```python
from build123d import *

# Parameters (mm, degrees)
F0_W      = 26
F0_H      = 26
F0_W_2    = 16
F0_H_2    = 16
F1_DEPTH  = 2
F2_DEPTH  = 100
F3_W      = 26
F3_H      = 26
F3_W_2    = 18
F3_H_2    = 18
F4_DEPTH  = 4
F5_W      = 5
F5_H      = 4
F6_DEPTH  = 4
F7_D      = 2.7
F7_DEPTH  = 4
F7_TIP    = 0.8111618357
F9_W      = 3
F9_H      = 16
F10_DEPTH = 26
F11_W     = 4
F11_H     = 12
F12_DEPTH = 20


with BuildPart() as f1:
    # F0 (on Top) → F1 (new body)
    with BuildSketch(Plane.XY):
        Rectangle(F0_W, F0_H)
        Rectangle(F0_W_2, F0_H_2, mode=Mode.SUBTRACT)
        Rectangle(F0_W_2, F0_H_2)
    extrude(amount=F1_DEPTH)

    # F0 (on Top) → F2 (join)
    with BuildSketch(Plane.XY):
        Rectangle(F0_W, F0_H)
        Rectangle(F0_W_2, F0_H_2, mode=Mode.SUBTRACT)
    extrude(amount=F2_DEPTH)

    # F3 (on face) → F4 (join)
    with BuildSketch(Plane.XY.offset(100)):
        Rectangle(F3_W, F3_H)
        Rectangle(F3_W_2, F3_H_2, mode=Mode.SUBTRACT)
    extrude(amount=F4_DEPTH)

    # F5 (on face) → F6 (cut, through all)
    with BuildSketch(Plane.XY.offset(104)):
        with Locations((0, -11)):
            Rectangle(F5_W, F5_H)
        with Locations((0, 11)):
            Rectangle(F5_W, F5_H)
    extrude(amount=-F6_DEPTH, mode=Mode.SUBTRACT)

    # F7
    with Locations(Plane.XY.offset(104)):
        with Locations((-10.5, 10.5), (10.5, 10.5), (-10.5, -10.5), (10.5, -10.5)):
            Hole(F7_D / 2, depth=F7_DEPTH)
            with Locations((0, 0, -(F7_DEPTH + F7_TIP / 2))):  # 118° drill point
                Cone(0, F7_D / 2, F7_TIP, mode=Mode.SUBTRACT)

    # F9 (on face) → F10 (join)
    with BuildSketch(Plane.XZ.offset(13)):
        with Locations((-14.5, 63)):
            Rectangle(F9_W, F9_H)
    extrude(amount=-F10_DEPTH)

    # F11 (on face) → F12 (cut)
    with BuildSketch(Plane.XZ.offset(13)):
        with Locations((-9, 63)):
            Rectangle(F11_W, F11_H)
    extrude(amount=-F12_DEPTH, mode=Mode.SUBTRACT)


solid = f1.part
```
Read the model definition and answer for the solid it produces. Units are mm, in the model's axes. A direction names the side the tool comes from. Round coordinates to 2 decimals unless told otherwise and drop trailing zeros. Write each loop counter-clockwise with the first axis right and the second up, starting at its lowest first coordinate (ties: lowest second). Pieces come first, ordered by that corner, then holes. Notation, with made-up numbers: M -33.75,83.5 L -10.75,83.5 A36 cw -10.75,120.5 Z; hole C 84.25,-20 d10. An arc over 180 degrees is marked long. One line per item, written item: value.
Q1. Flat-ended cylindrical pins translate along their axes: pin 1 Ø1.6 at (x, y) = (10.5, -10.5) entering from -Z; pin 2 Ø3 at (y, z) = (11.5, 102.5) entering from -X; pin 3 Ø1.5 at (x, y) = (-15, 2.5) entering from -Z; pin 4 Ø0.9 at (x, y) = (-15, 0.5) entering from +Z. Find the tip coordinate at first contact, or state that the pin passes through.
Data:
pin 1: z = 0
pin 2: x = -13
pin 3: z = 55
pin 4: z = 71
Q2. Find section B-B on z = 16. Write down the section's boundary in (x, y), plus the area to 3 significant figures.
Data:
outline: M -13,-13 L 13,-13 L 13,13 L -13,13 Z; hole M -8,-8 L 8,-8 L 8,8 L -8,8 Z
area: 420 mm2
Q3. Find section C-C on x = 3.75. Write down the section's boundary in (y, z).
Data:
outline: M -13,0 L 13,0 L 13,104 L 9,104 L 9,100 L 8,100 L 8,2 L -8,2 L -8,100 L -9,100 L -9,104 L -13,104 Z
Q4. Find section A-A on y = -2.5. Write down the section's boundary in (x, z).
Data:
outline: M -16,55 L -13,55 L -13,0 L 13,0 L 13,104 L 9,104 L 9,100 L 8,100 L 8,2 L -8,2 L -8,57 L -11,57 L -11,69 L -8,69 L -8,100 L -9,100 L -9,104 L -13,104 L -13,71 L -16,71 Z
Q5. Which of the six approach directions +Z, -Z, +X, -X, +Y, -Y give full straight-line access (tool end or side, diameter ignored) to faces 1 (the flat face through (-13, 0, 87)), 2 (the flat face through (-9, -3, 57)), 3 (the flat face through (0, 8, 50)), 4 (the flat face through (-16, 0, 63))?
Data:
face 1: +Z, -X, +Y, -Y
face 2: -Y
face 3: +Z
face 4: +Z, -Z, -X, +Y, -Y
Q6. Straight lines are drawn through the part: line 1 (X direction, y = -10.5, z = 102.65); line 2 (Y direction, x = -10.5, z = 101.35); line 3 (X direction, y = 7.75, z = 20.5). For each, find the intervals that lie inside material, in ascending order. Write a range as [from, to].
Data:
line 1: [-13, -11.85], [-9.15, -2.5], [2.5, 9.15], [11.85, 13]
line 2: [-13, -11.85], [-9.15, 9.15], [11.85, 13]
line 3: [-13, -8], [8, 13]
Q7. For a pull along Z with two mould halves and no side action, classify faces 5 (the flat face through (-2, 13, 51)), 6 (the conical face through (-10.28, -10.59, 99.33)), 7 (the flat face through (-11, -3, 63)) as +Z half, -Z half, draft (parallel to the pull), parting line (faces both ways), or undercut.
Data:
face 5: draft
face 6: +Z half
face 7: undercut
